Model file for the job. Use its own axes, mm. Face numbers are marked on the shaded views. A direction names the side the tool comes from. Round coordinates to 2 decimals unless told otherwise and drop trailing zeros. Loops run counter-clockwise (first coordinate to the right, second up) from the corner with the lowest first, then second, coordinate; pieces in that order, holes last. Notation, with made-up numbers: (-16.5, -16.75) - (29.5, -16.75) arc R25 ccw to (29.5, 2.25) - close; hole circle Ø8 at (34, 81). An arc over 180 degrees is marked (long way). Use one line per item in the form item = value.
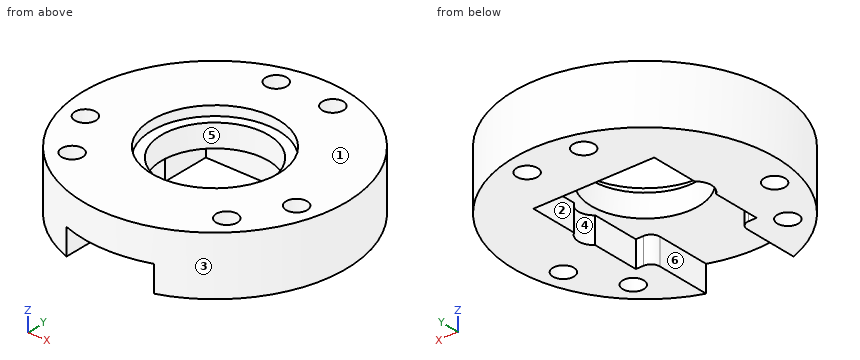
from build123d import *

# Parameters (mm, degrees)
EXTRUDE_1_DEPTH     = 3
CUT_EXTRUDE_4_DEPTH = 22.424285286
SKETCH_12_R         = 15
SKETCH_12_R_2       = 6.125
EXTRUDE_2_DEPTH     = 2.6
SKETCH_13_R         = 15
SKETCH_13_R_2       = 7.25
EXTRUDE_3_DEPTH     = 1.1
SKETCH_14_R         = 1.2
CUT_EXTRUDE_5_DEPTH = 23.246123258
FILLET_1_R          = 1


with BuildPart() as part:
    # 스케치1 → 보스-돌출1 (new body)
    with BuildSketch(Plane.XY):
        with BuildLine():
            Line((-5, -6.9), (-6.9, -6.9))
            Line((-6.9, -6.9), (-6.9, 6.9))
            Line((-6.9, 6.9), (6.9, 6.9))
            Line((6.9, 6.9), (6.9, -6.9))
            Line((6.9, -6.9), (5, -6.9))
            Line((5, -6.9), (5, -14.142135624))
            ThreePointArc((5, -14.142135624), (0, 15), (-5, -14.142135624))
            Line((-5, -14.142135624), (-5, -6.9))
        make_face()
    extrude(amount=EXTRUDE_1_DEPTH)

    # 스케치11 → 컷-돌출4 (cut, through all)
    with BuildSketch(Plane.XY.offset(3)):
        with BuildLine():
            Line((5.8, -1.8), (-5.8, -1.8))
            ThreePointArc((-5.8, -1.8), (-7.6, 0), (-5.8, 1.8))
            Line((-5.8, 1.8), (5.8, 1.8))
            ThreePointArc((5.8, 1.8), (7.6, 0), (5.8, -1.8))
        make_face()
    extrude(amount=-CUT_EXTRUDE_4_DEPTH, mode=Mode.SUBTRACT)

    # 스케치12 → 보스-돌출2 (add)
    with BuildSketch(Plane.XY.offset(3)):
        with Locations(Location((0, 0, 0), (0, 0, 250.528779366))):
            Circle(SKETCH_12_R)
        Circle(SKETCH_12_R_2, mode=Mode.SUBTRACT)
    extrude(amount=EXTRUDE_2_DEPTH)

    # 스케치13 → 보스-돌출3 (add)
    with BuildSketch(Plane.XY.offset(5.6)):
        with Locations(Location((0, 0, 0), (0, 0, 250.528779366))):
            Circle(SKETCH_13_R)
        Circle(SKETCH_13_R_2, mode=Mode.SUBTRACT)
    extrude(amount=EXTRUDE_3_DEPTH)

    # 스케치14 → 컷-돌출5 (cut, through all)
    with BuildSketch(Plane.XY.offset(6.7)):
        with Locations((3.235238064, 12.074072829)):
            Circle(SKETCH_14_R)
        with Locations((-3.235238064, 12.074072829)):
            Circle(SKETCH_14_R)
        with Locations((12.074072829, -3.235238064)):
            Circle(SKETCH_14_R)
        with Locations((8.838834765, -8.838834765)):
            Circle(SKETCH_14_R)
        with Locations((-8.838834765, -8.838834765)):
            Circle(SKETCH_14_R)
        with Locations((-12.074072829, -3.235238064)):
            Circle(SKETCH_14_R)
    extrude(amount=-CUT_EXTRUDE_5_DEPTH, mode=Mode.SUBTRACT)

    # 필렛1
    fillet_1_edges = [part.edges().sort_by_distance(p)[0] for p in [
        (-5, -6.9, 1.5),
        (5, -6.9, 1.5),
    ]]
    fillet(fillet_1_edges, radius=FILLET_1_R)


solid = part.part
1. Flat gauge pins, fed straight in: pin 1 (0.7 mm diameter, centred on x = 6.5, z = 1.5, fed in from +Y); pin 2 (3.5 mm diameter, centred on y = -11.5, z = 2, fed in from +X); pin 3 (8 mm diameter, centred on x = -1, y = -0.5, fed in from +Z); pin 4 (0.9 mm diameter, centred on y = -3, z = 1.5, fed in from -X). Where does each tip first touch, or does it go through?
Geometry check:
pin_1 = 13.68
pin_2 = 11.4
pin_3 = through
pin_4 = -14.78
2. Tool access for the marked faces 4, 5 and 6: list every direction of +Z, -Z, +X, -X, +Y, -Y with a clear straight run to the whole face (end or side of a thin tool).
Geometry check:
face_4 = -Z
face_5 = +Z, -Z
face_6 = -Z, -Y
3. Cut at C-C, the plane z = 1. Give the cut face in (x, y), plus the area to 3 significant figures.
Geometry check:
outline = (-6.9, -6.9) - (-6.9, -1.42) arc R1.8 cw to (-6.9, 1.42) - (-6.9, 6.9) - (6.9, 6.9) - (6.9, 1.42) arc R1.8 cw to (6.9, -1.42) - (6.9, -6.9) - (6, -6.9) arc R1 ccw to (5, -7.9) - (5, -14.14) arc R15 ccw (long way) to (-5, -14.14) - (-5, -7.9) arc R1 ccw to (-6, -6.9) - close; hole circle Ø2.4 at (-12.07, -3.24); hole circle Ø2.4 at (-8.84, -8.84); hole circle Ø2.4 at (-3.24, 12.07); hole circle Ø2.4 at (3.24, 12.07); hole circle Ø2.4 at (8.84, -8.84); hole circle Ø2.4 at (12.07, -3.24)
area = 408 mm^2
4. Cut at B-B, the plane y = 0. Give the cut face in (x, z) (3 decimals), plus the area to 3 significant figures.
Geometry check:
outline = (-15, 0) - (-7.6, 0) - (-7.6, 3) - (-6.125, 3) - (-6.125, 5.6) - (-7.25, 5.6) - (-7.25, 6.7) - (-15, 6.7) - close; (6.125, 3) - (7.6, 3) - (7.6, 0) - (15, 0) - (15, 6.7) - (7.25, 6.7) - (7.25, 5.6) - (6.125, 5.6) - close
area = 108 mm^2
5. Cut at D-D, the plane z = 6. Give the cut face in (x, y), plus the area to 3 significant figures.
Geometry check:
outline = circle Ø30 at (0, 0); hole circle Ø2.4 at (-12.07, -3.24); hole circle Ø2.4 at (-8.84, -8.84); hole circle Ø14.5 at (0, 0); hole circle Ø2.4 at (-3.24, 12.07); hole circle Ø2.4 at (3.24, 12.07); hole circle Ø2.4 at (8.84, -8.84); hole circle Ø2.4 at (12.07, -3.24)
area = 515 mm^2
6. Wall check: probe 1 along X at (y, z) = (-2.75, 2.75); probe 2 along X at (y, z) = (0.25, 4.75); probe 3 along X at (y, z) = (-8.5, 6.25). Give the ranges that are in metal, low to high.
Geometry check:
probe_1 = -14.75 to -13.17, -10.98 to -6.9, 6.9 to 10.98, 13.17 to 14.75
probe_2 = -15 to -6.12, 6.12 to 15
probe_3 = -12.36 to -9.99, -7.69 to 7.69, 9.99 to 12.36
7. Pull direction X, two halves, no side cores. Call the marked faces 1, 2 and 3: +X half, -X half, draft (parallel to the pull), parting line (faces both ways), or undercut.
Geometry check:
face_1 = draft
face_2 = undercut
face_3 = parting line
8. Cut at A-A, the plane x = 0. Give the cut face in (y, z) (3 decimals).
Geometry check:
outline = (-15, 3) - (-6.125, 3) - (-6.125, 5.6) - (-7.25, 5.6) - (-7.25, 6.7) - (-15, 6.7) - close; (6.125, 3) - (6.9, 3) - (6.9, 0) - (15, 0) - (15, 6.7) - (7.25, 6.7) - (7.25, 5.6) - (6.125, 5.6) - close
